```python
from build123d import *

# Parameters (mm, degrees)
SKETCH_1_W          = 105
SKETCH_1_H          = 105
SKETCH_1_R          = 2.75
SKETCH_1_W_2        = 81
SKETCH_1_H_2        = 81
SKETCH_1_R_2        = 1.4
EXTRUDE_1_DEPTH     = 4
EXTRUDE_START       = 4
SKETCH_1_4_R        = 2.75
SKETCH_1_4_R_2      = 1.4
EXTRUDE_2_DEPTH     = 2
EXTRUDE_START_2     = -25
EXTRUDE_3_DEPTH     = 55
CUT_EXTRUDE_1_REACH = 97.836
SKETCH_3_R          = 2.2
FILLET_1_R          = 3
FILLET_2_R          = 10


with BuildPart() as part:
    # 草图1 → 凸台-拉伸1 (new body)
    # profile 1 of 5: a face of its own
    with BuildSketch(Plane(origin=(0, 0, 0), x_dir=(1, 0, 0), z_dir=(0, 1, 0))):
        Rectangle(SKETCH_1_W, SKETCH_1_H)
        with Locations((46, 46)):
            Circle(SKETCH_1_R, mode=Mode.SUBTRACT)
        with Locations((-46, 46)):
            Circle(SKETCH_1_R, mode=Mode.SUBTRACT)
        with Locations((46, -46)):
            Circle(SKETCH_1_R, mode=Mode.SUBTRACT)
        with Locations((-46, -46)):
            Circle(SKETCH_1_R, mode=Mode.SUBTRACT)
        Rectangle(SKETCH_1_W_2, SKETCH_1_H_2, mode=Mode.SUBTRACT)
    # profile 2 of 5: a face of its own
    with BuildSketch(Plane(origin=(0, 0, 0), x_dir=(1, 0, 0), z_dir=(0, 1, 0))):
        with Locations((46, 46)):
            Circle(SKETCH_1_R)
        with Locations(Location((46, 46, 0), (0, 0, 270))):
            Circle(SKETCH_1_R_2, mode=Mode.SUBTRACT)
    # profile 3 of 5: a face of its own
    with BuildSketch(Plane(origin=(0, 0, 0), x_dir=(1, 0, 0), z_dir=(0, 1, 0))):
        with Locations((-46, 46)):
            Circle(SKETCH_1_R)
        with Locations(Location((-46, 46, 0), (0, 0, 270))):
            Circle(SKETCH_1_R_2, mode=Mode.SUBTRACT)
    # profile 4 of 5: a face of its own
    with BuildSketch(Plane(origin=(0, 0, 0), x_dir=(1, 0, 0), z_dir=(0, 1, 0))):
        with Locations((-46, -46)):
            Circle(SKETCH_1_R)
        with Locations(Location((-46, -46, 0), (0, 0, 270))):
            Circle(SKETCH_1_R_2, mode=Mode.SUBTRACT)
    # profile 5 of 5: a face of its own
    with BuildSketch(Plane(origin=(0, 0, 0), x_dir=(1, 0, 0), z_dir=(0, 1, 0))):
        with Locations((46, -46)):
            Circle(SKETCH_1_R)
        with Locations(Location((46, -46, 0), (0, 0, 270))):
            Circle(SKETCH_1_R_2, mode=Mode.SUBTRACT)
    extrude(amount=EXTRUDE_1_DEPTH)

    # 草图1<4> → 凸台-拉伸2 (add)
    # profile 1 of 4: a face of its own
    with BuildSketch(Plane(origin=(0, 0, 0), x_dir=(1, 0, 0), z_dir=(0, 1, 0)).offset(EXTRUDE_START)):
        with Locations(Location((-46, 46, 0), (0, 0, 270))):
            Circle(SKETCH_1_4_R)
        with Locations(Location((-46, 46, 0), (0, 0, 270))):
            Circle(SKETCH_1_4_R_2, mode=Mode.SUBTRACT)
    # profile 2 of 4: a face of its own
    with BuildSketch(Plane(origin=(0, 0, 0), x_dir=(1, 0, 0), z_dir=(0, 1, 0)).offset(EXTRUDE_START)):
        with Locations(Location((46, 46, 0), (0, 0, 270))):
            Circle(SKETCH_1_4_R)
        with Locations(Location((46, 46, 0), (0, 0, 270))):
            Circle(SKETCH_1_4_R_2, mode=Mode.SUBTRACT)
    # profile 3 of 4: a face of its own
    with BuildSketch(Plane(origin=(0, 0, 0), x_dir=(1, 0, 0), z_dir=(0, 1, 0)).offset(EXTRUDE_START)):
        with Locations(Location((46, -46, 0), (0, 0, 270))):
            Circle(SKETCH_1_4_R)
        with Locations(Location((46, -46, 0), (0, 0, 270))):
            Circle(SKETCH_1_4_R_2, mode=Mode.SUBTRACT)
    # profile 4 of 4: a face of its own
    with BuildSketch(Plane(origin=(0, 0, 0), x_dir=(1, 0, 0), z_dir=(0, 1, 0)).offset(EXTRUDE_START)):
        with Locations(Location((-46, -46, 0), (0, 0, 270))):
            Circle(SKETCH_1_4_R)
        with Locations(Location((-46, -46, 0), (0, 0, 270))):
            Circle(SKETCH_1_4_R_2, mode=Mode.SUBTRACT)
    extrude(amount=EXTRUDE_2_DEPTH)

    # 草图2 → 凸台-拉伸3 (add)
    with BuildSketch(Plane.ZY.offset(52.5).offset(EXTRUDE_START_2)):
        Polygon((52.5, 0), (56.5, 0), (56.5, 20), (76.5, 20), (76.5, 24), (52.5, 24), align=None)
    extrude(amount=-EXTRUDE_3_DEPTH)

    # 草图3 → 切除-拉伸1 (cut, up to next)
    with BuildSketch(Plane(origin=(0, 24, 0), x_dir=(1, 0, 0), z_dir=(0, 1, 0)), mode=Mode.PRIVATE) as cut_extrude_1_sk1:
        with Locations(Location((17.5, -66.5, 0), (0, 0, 270))):
            Circle(SKETCH_3_R)
    cut_extrude_1_tool1 = extrude(cut_extrude_1_sk1.sketch, amount=-CUT_EXTRUDE_1_REACH, mode=Mode.PRIVATE) & part.part
    # 草图3 → 切除-拉伸1 (cut, up to next)
    with BuildSketch(Plane(origin=(0, 24, 0), x_dir=(1, 0, 0), z_dir=(0, 1, 0)), mode=Mode.PRIVATE) as cut_extrude_1_sk2:
        with Locations(Location((-17.5, -66.5, 0), (0, 0, 270))):
            Circle(SKETCH_3_R)
    cut_extrude_1_tool2 = extrude(cut_extrude_1_sk2.sketch, amount=-CUT_EXTRUDE_1_REACH, mode=Mode.PRIVATE) & part.part
    add(cut_extrude_1_tool1.solids().sort_by_distance((17.5, 24, 66.5))[0], mode=Mode.SUBTRACT)
    add(cut_extrude_1_tool2.solids().sort_by_distance((-17.5, 24, 66.5))[0], mode=Mode.SUBTRACT)

    # 圆角1
    fillet_1_edges = [part.edges().sort_by_distance(p)[0] for p in [
        (-52.5, 2, -52.5),
        (52.5, 2, -52.5),
        (52.5, 2, 52.5),
        (27.5, 22, 76.5),
        (-27.5, 22, 76.5),
        (-52.5, 2, 52.5),
    ]]
    fillet(fillet_1_edges, radius=FILLET_1_R)

    # 圆角2
    # the kernel refuses this fillet: 10 mm, written as the material it adds along each edge
    with BuildSketch(Plane(origin=(27.5, 4, 52.5), x_dir=(1, 0, 0), z_dir=(0, -1, 0))) as fillet_2_piece_1:
        with BuildLine():
            CenterArc((8, 10), FILLET_2_R, 216.869897646, 53.130102354)
            Line((0, 4), (0, 0))
            Line((0, 0), (8, 0))
        make_face()
    extrude(amount=4)
    with BuildSketch(Plane(origin=(-27.5, 4, 52.5), x_dir=(0, 0, 1), z_dir=(0, -1, 0))) as fillet_2_piece_2:
        with BuildLine():
            CenterArc((10, 8), FILLET_2_R, 180, 53.130102354)
            Line((0, 8), (0, 0))
            Line((0, 0), (4, 0))
        make_face()
    extrude(amount=4)


solid = part.part
```
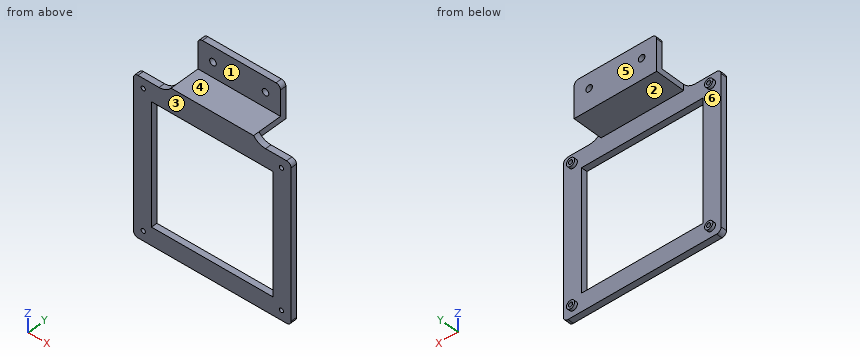
For this review, take the finished solid that the model builds, in its own axes (mm). Face numbers are marked on the shaded views. A direction names the side the tool comes from. Round coordinates to 2 decimals unless told otherwise and drop trailing zeros. Write each loop counter-clockwise with the first axis right and the second up, starting at its lowest first coordinate (ties: lowest second). Pieces come first, ordered by that corner, then holes. Notation, with made-up numbers: (-36.75, 88) - (-8.75, 88) arc R25 ccw to (-8.75, 121) - close; hole circle Ø1 at (70.5, 38.5). An arc over 180 degrees is marked (long way). Answer as CSV lines item,"result". Start each with the question number.
(1) Machinability: for the marked faces 1, 2 and 3, which of the approach directions +Z, -Z, +X, -X, +Y, -Y give a long, thin tool a straight path to every point of the face, cutting with its end or side? Answer none if there is none.
(2) Add section D-D, the plane z = 21.5. State the section outline as (x, y) points.
(3) For pin 1 (3 mm diameter, centred on x = 11.5, y = 5, fed in from +Z); pin 2 (3 mm diameter, centred on x = 41, y = 2, fed in from +Z); pin 3 (6 mm diameter, centred on x = 45, z = -47.5, fed in from +Y), all flat-tipped, find the tip position at first contact; note any pin that passes through.
(4) Mouldability with a two-part tool opening along Z and no side actions: class the marked faces 4, 5 and 6 as +Z half, -Z half, draft (parallel to the pull), parting line (faces both ways), or undercut.
(5) Add section B-B, the plane z = 66.5. State the section outline as (x, y) points, plus the area to 3 significant figures.
(6) Add section A-A, the plane x = -17.5. State the section outline as (y, z) points.
(7) For line 1 (X direction, y = 2.75, z = 46); line 2 (X direction, y = 22.05, z = 66.5); line 3 (Z direction, x = 11, y = 7), list the stretches that pass through material, from the lowest coordinate up.
(8) Add section C-C, the plane y = 2.5. State the section outline as (x, z) points.
From the geometry:
1,face 1,"+Z, +X, -X, -Y"
1,face 2,"-Z, +X, -X, +Y"
1,face 3,"+Z, -Z, +X, -X, -Y"
2,outline,"(-52.5, 0) - (-40.5, 0) - (-40.5, 4) - (-52.5, 4) - close; (40.5, 0) - (52.5, 0) - (52.5, 4) - (40.5, 4) - close"
3,pin 1,"stops at z = 56.5"
3,pin 2,"stops at z = 52.5"
3,pin 3,"stops at y = 6"
4,face 4,"+Z half"
4,face 5,"draft"
4,face 6,"undercut"
5,outline,"(-27.5, 20) - (-19.7, 20) - (-19.7, 24) - (-27.5, 24) - close; (-15.3, 20) - (15.3, 20) - (15.3, 24) - (-15.3, 24) - close; (19.7, 20) - (27.5, 20) - (27.5, 24) - (19.7, 24) - close"
5,area,"185 mm²"
6,outline,"(0, -52.5) - (4, -52.5) - (4, -40.5) - (0, -40.5) - close; (0, 40.5) - (4, 40.5) - (4, 52.5) - (24, 52.5) - (24, 64.3) - (20, 64.3) - (20, 56.5) - (0, 56.5) - close; (20, 68.7) - (24, 68.7) - (24, 76.5) - (20, 76.5) - close"
7,line 1,"x = -52.5 to -47.4, -44.6 to 44.6, 47.4 to 52.5"
7,line 2,"x = -27.5 to -19.7, -15.3 to 15.3, 19.7 to 27.5"
7,line 3,"z = 52.5 to 56.5"
8,outline,"(-52.5, -49.5) arc R3 ccw to (-49.5, -52.5) - (49.5, -52.5) arc R3 ccw to (52.5, -49.5) - (52.5, 49.5) arc R3 ccw to (49.5, 52.5) - (35.5, 52.5) arc R10 cw to (27.5, 56.5) - (-27.5, 56.5) arc R10 cw to (-35.5, 52.5) - (-49.5, 52.5) arc R3 ccw to (-52.5, 49.5) - close; hole circle Ø2.8 at (-46, -46); hole circle Ø2.8 at (-46, 46); hole (-40.5, -40.5) - (40.5, -40.5) - (40.5, 40.5) - (-40.5, 40.5) - close; hole circle Ø2.8 at (46, -46); hole circle Ø2.8 at (46, 46)"
